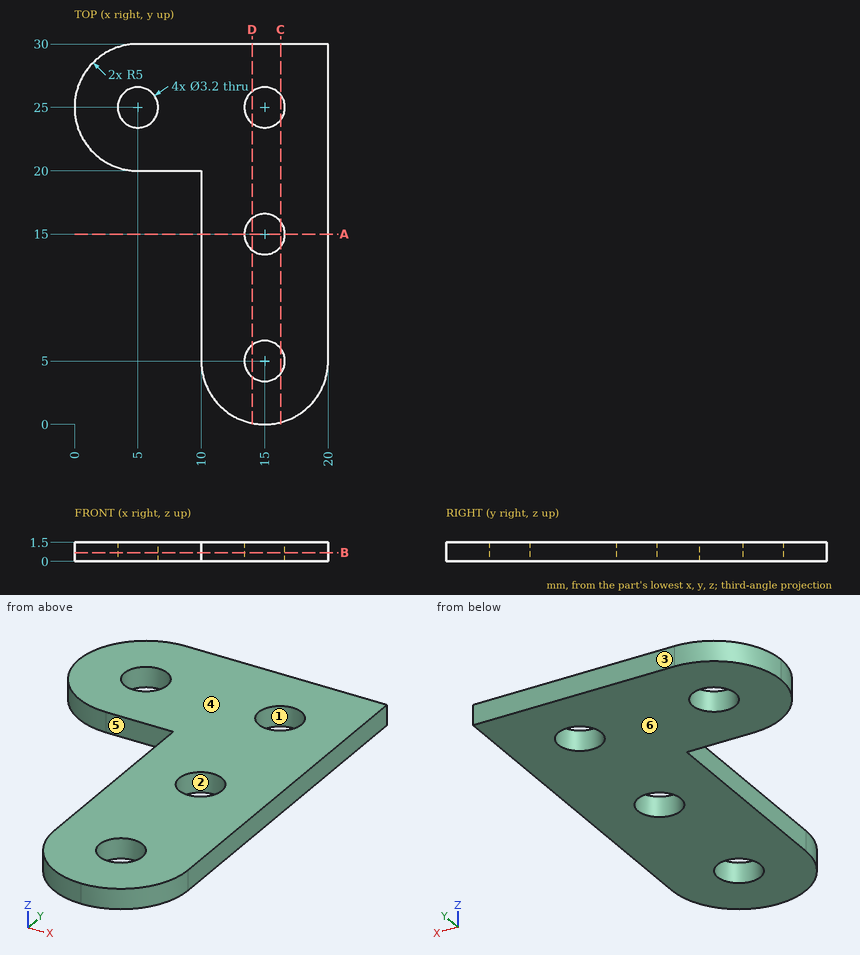
Source: three-view drawing plus pictorial views. Frame: mm from the lowest corner of the part. A direction names the side the tool comes from. Coordinates: 2 decimals unless noted, no trailing zeros. Order: outer loops, then holes, each group sorted by start corner. A loop starts at its lowest first (then second) coordinate and runs counter-clockwise, first axis right, second up.
1) Set-up query: the marked faces 5 and 6. Return all of +Z, -Z, +X, -X, +Y, -Y with unobstructed straight access to the full face (end or side cutting, diameter ignored); none if empty.
Result sheet:
face 5: +Z, -Z, -X, -Y
face 6: -Z, +X, -X, +Y, -Y
2) Section B-B (z = 0.7). Return loops of the section in (x, y), then the cut area to 3 significant figures.
Result sheet:
outline: (5, 20) - (10, 20) - (10, 5) arc R5 ccw to (20, 5) - (20, 30) - (5, 30) arc R5 ccw to start; hole circle Ø3.2 at (5, 25); hole circle Ø3.2 at (15, 5); hole circle Ø3.2 at (15, 15); hole circle Ø3.2 at (15, 25)
area: 346 mm2
3) First-contact query: P1, Ø1.9, axis at x = 15, y = 25, coming from the +Z side. Flat tip, straight axial feed; report the tip coordinate or a pass-through.
Result sheet:
P1: passes through
4) Ray query, probe 1 along Y at (x, z) = (15.75, 0.75); probe 2 along Y at (x, z) = (14, 0.95); probe 3 along X at (y, z) = (9, 1.3). Return the intervals inside material, ascending.
Result sheet:
probe 1: y = 0.06 to 3.59, 6.41 to 13.59, 16.41 to 23.59, 26.41 to 30
probe 2: y = 0.1 to 3.75, 6.25 to 13.75, 16.25 to 23.75, 26.25 to 30
probe 3: x = 10 to 20
5) Draft query along Y for the marked faces 1, 2, 3 and 4. Return one class per face: released by +Y, released by -Y, zero draft, split by the parting line, or undercut.
Result sheet:
face 1: undercut
face 2: undercut
face 3: released by +Y
face 4: zero draft
6) Section C-C (x = 16.25). Return loops of the section in (y, z), then the cut area to 3 significant figures.
Result sheet:
outline: (0.16, 0) - (4, 0) - (4, 1.5) - (0.16, 1.5) - close; (6, 0) - (14, 0) - (14, 1.5) - (6, 1.5) - close; (16, 0) - (24, 0) - (24, 1.5) - (16, 1.5) - close; (26, 0) - (30, 0) - (30, 1.5) - (26, 1.5) - close
area: 35.8 mm2
7) Section D-D (x = 14). Return loops of the section in (y, z).
Result sheet:
outline: (0.1, 0) - (3.75, 0) - (3.75, 1.5) - (0.1, 1.5) - close; (6.25, 0) - (13.75, 0) - (13.75, 1.5) - (6.25, 1.5) - close; (16.25, 0) - (23.75, 0) - (23.75, 1.5) - (16.25, 1.5) - close; (26.25, 0) - (30, 0) - (30, 1.5) - (26.25, 1.5) - close
8) Section A-A (y = 15). Return loops of the section in (x, z), then the cut area to 3 significant figures.
Result sheet:
outline: (10, 0) - (13.4, 0) - (13.4, 1.5) - (10, 1.5) - close; (16.6, 0) - (20, 0) - (20, 1.5) - (16.6, 1.5) - close
area: 10.2 mm2
